Build history of the part. All positions in model axes, mm. A direction names the side the tool comes from. Round coordinates to 2 decimals unless told otherwise and drop trailing zeros. Write each loop counter-clockwise with the first axis right and the second up, starting at its lowest first coordinate (ties: lowest second). Pieces come first, ordered by that corner, then holes.
Item 1: Band-saw the part on C-C, the plane y = 12. Write the cut outline in (x, z).
Item 2: Band-saw the part on D-D, the plane y = 18. Write the cut outline in (x, z), then the cut area to 3 significant figures.
Item 3: Mould opens along Z. For faces 3 (the cylindrical face through (11.14, 0.59, 10.06)), 4 (the cylindrical face through (-2.61, 43.75, 8.3)), 5 (the flat face through (-6, 0, 0)) say: +Z half, -Z half, draft (parallel to the pull), parting line (faces both ways), or undercut.
Item 4: Drop flat-ended pins along their axis: pin 1 Ø2 at (x, z) = (14.85, -14.85) entering from -Y; pin 2 Ø3 at (x, z) = (0, -19.8) entering from +Y; pin 3 Ø2 at (x, z) = (-4.95, 14.85) entering from -Y; pin 4 Ø1.5 at (x, z) = (-4.95, 4.95) entering from +Y. Give the stop position or say it passes through.
Item 5: Wall check: probe 1 along X at (y, z) = (42, 0.5); probe 2 along X at (y, z) = (10.5, -14.5); probe 3 along Z at (x, y) = (7, 31.5). Give the ranges that are in metal, low to high.
Item 6: Band-saw the part on A-A, the plane x = 0. Count the separate pieces of the cut face and the enclosed holes in it, then the cut area to 3 significant figures.
Item 7: 3-axis set-ups, long thin cutter, end or side, ignore diameter. For faces 1 (the cylindrical face through (18.58, 0.59, 10.17)), 2 (the cylindrical face through (-1.22, 0.59, 0.27)): which of +Z, -Z, +X, -X, +Y, -Y reach the whole face in a straight line?
```python
from build123d import *

# Parameters (mm, degrees)
ESQUISSE3_R             = 1.25
ENL_V_MAT_EXTRU_2_DEPTH = 1.2
CONG_1_R                = 15


with BuildPart() as part:
    # Esquisse2 → Révolution1 (revolve)
    with BuildSketch(Plane(origin=(0, 0, 0), x_dir=(0, 0, -1), z_dir=(1, 0, 0)), mode=Mode.PRIVATE) as r_volution1_sk:
        with BuildLine():
            Line((8.7, 31.566988195), (26.843493008, 4.67800089))
            ThreePointArc((26.843493008, 4.67800089), (27.005627419, 1.591810146), (24.356665106, 0))
            Line((24.356665106, 0), (0, 0))
            Line((0, 0), (0, 1.2))
            Line((0, 1.2), (24.356665106, 1.2))
            ThreePointArc((24.356665106, 1.2), (25.946042494, 2.155086088), (25.848761847, 4.006800534))
            Line((25.848761847, 4.006800534), (7.5, 31.2))
            Line((7.5, 31.2), (7.5, 51.566988195))
            Line((7.5, 51.566988195), (8.7, 51.566988195))
            Line((8.7, 51.566988195), (8.7, 31.566988195))
        make_face()
    revolve(r_volution1_sk.sketch.rotate(Axis((0, 1.2, 0), (0, -1, 0)), 180), axis=Axis((0, 1.2, 0), (0, -1, 0)))

    # Esquisse3 → Enlèv. mat.-Extru.2 (cut)
    with BuildSketch(Plane.XZ):
        with Locations(Location((-9.899494937, 0, 0), (0, 0, 270))):
            Circle(ESQUISSE3_R)
        with Locations(Location((-4.949747468, -4.949747468, 0), (0, 0, 270))):
            Circle(ESQUISSE3_R)
        with Locations(Location((0, 0, 0), (0, 0, 270))):
            Circle(ESQUISSE3_R)
        with Locations(Location((4.949747468, 4.949747468, 0), (0, 0, 270))):
            Circle(ESQUISSE3_R)
        with Locations(Location((9.899494937, 19.798989873, 0), (0, 0, 270))):
            Circle(ESQUISSE3_R)
        with Locations(Location((4.949747468, 14.849242405, 0), (0, 0, 270))):
            Circle(ESQUISSE3_R)
        with Locations(Location((14.849242405, 14.849242405, 0), (0, 0, 270))):
            Circle(ESQUISSE3_R)
        with Locations(Location((19.798989873, 9.899494937, 0), (0, 0, 270))):
            Circle(ESQUISSE3_R)
        with Locations(Location((14.849242405, 4.949747468, 0), (0, 0, 270))):
            Circle(ESQUISSE3_R)
        with Locations(Location((19.798989873, 0, 0), (0, 0, 270))):
            Circle(ESQUISSE3_R)
        with Locations(Location((14.849242405, -4.949747468, 0), (0, 0, 270))):
            Circle(ESQUISSE3_R)
        with Locations(Location((-19.798989873, 0, 0), (0, 0, 270))):
            Circle(ESQUISSE3_R)
        with Locations(Location((-14.849242405, 4.949747468, 0), (0, 0, 270))):
            Circle(ESQUISSE3_R)
        with Locations(Location((-19.798989873, 9.899494937, 0), (0, 0, 270))):
            Circle(ESQUISSE3_R)
        with Locations(Location((-14.849242405, 14.849242405, 0), (0, 0, 270))):
            Circle(ESQUISSE3_R)
        with Locations(Location((-9.899494937, 19.798989873, 0), (0, 0, 270))):
            Circle(ESQUISSE3_R)
        with Locations(Location((0, 19.798989873, 0), (0, 0, 270))):
            Circle(ESQUISSE3_R)
        with Locations(Location((-4.949747468, 14.849242405, 0), (0, 0, 270))):
            Circle(ESQUISSE3_R)
        with Locations(Location((-9.899494937, 9.899494937, 0), (0, 0, 270))):
            Circle(ESQUISSE3_R)
        with Locations(Location((-4.949747468, 4.949747468, 0), (0, 0, 270))):
            Circle(ESQUISSE3_R)
        with Locations(Location((0, 9.899494937, 0), (0, 0, 270))):
            Circle(ESQUISSE3_R)
        with Locations(Location((9.899494937, 9.899494937, 0), (0, 0, 270))):
            Circle(ESQUISSE3_R)
        with Locations(Location((9.899494937, 0, 0), (0, 0, 270))):
            Circle(ESQUISSE3_R)
        with Locations(Location((4.949747468, -4.949747468, 0), (0, 0, 270))):
            Circle(ESQUISSE3_R)
        with Locations(Location((0, -9.899494937, 0), (0, 0, 270))):
            Circle(ESQUISSE3_R)
        with Locations(Location((-9.899494937, -9.899494937, 0), (0, 0, 270))):
            Circle(ESQUISSE3_R)
        with Locations(Location((-14.849242405, -4.949747468, 0), (0, 0, 270))):
            Circle(ESQUISSE3_R)
        with Locations(Location((-19.798989873, -9.899494937, 0), (0, 0, 270))):
            Circle(ESQUISSE3_R)
        with Locations(Location((-14.849242405, -14.849242405, 0), (0, 0, 270))):
            Circle(ESQUISSE3_R)
        with Locations(Location((-9.899494937, -19.798989873, 0), (0, 0, 270))):
            Circle(ESQUISSE3_R)
        with Locations(Location((-4.949747468, -14.849242405, 0), (0, 0, 270))):
            Circle(ESQUISSE3_R)
        with Locations(Location((0, -19.798989873, 0), (0, 0, 270))):
            Circle(ESQUISSE3_R)
        with Locations(Location((4.949747468, -14.849242405, 0), (0, 0, 270))):
            Circle(ESQUISSE3_R)
        with Locations(Location((9.899494937, -9.899494937, 0), (0, 0, 270))):
            Circle(ESQUISSE3_R)
        with Locations(Location((9.899494937, -19.798989873, 0), (0, 0, 270))):
            Circle(ESQUISSE3_R)
        with Locations(Location((14.849242405, -14.849242405, 0), (0, 0, 270))):
            Circle(ESQUISSE3_R)
        with Locations(Location((19.798989873, -9.899494937, 0), (0, 0, 270))):
            Circle(ESQUISSE3_R)
    extrude(amount=-ENL_V_MAT_EXTRU_2_DEPTH, mode=Mode.SUBTRACT)

    # Congé1
    cong_1_edges = [part.edges().sort_by_distance(p)[0] for p in [
        (0, 31.566988195, -8.7),
        (0, 31.2, -7.5),
    ]]
    fillet(cong_1_edges, radius=CONG_1_R)


solid = part.part
```
Results:
1. outline: circle Ø43.81 at (0, 0); hole circle Ø40.91 at (0, 0)
2. outline: circle Ø35.71 at (0, 0); hole circle Ø32.81 at (0, 0)
2. area: 156 mm2
3. face 3: undercut
3. face 4: parting line
3. face 5: draft
4. pin 1: stops at y = 9.71
4. pin 2: stops at y = 17.34
4. pin 3: stops at y = 17.63
4. pin 4: stops at y = 51.57
5. probe 1: x = -8.69 to -7.48, 7.48 to 8.69
5. probe 2: x = -17.74 to -15.83, 15.83 to 17.74
5. probe 3: z = -6.33 to -4.13, 4.13 to 6.33
6. separate pieces: 6
6. enclosed holes: 0
6. area: 183 mm2
7. face 1: -Y
7. face 2: +Y, -Y
